The model under review builds one solid part; all positions refer to its coordinate system, in mm. A direction names the side the tool comes from. Give positions to 0.01 mm unless a question says otherwise; leave off trailing zeros. Write each loop counter-clockwise with the first axis right and the second up, starting at its lowest first coordinate (ties: lowest second). Pieces come first, ordered by that corner, then holes. Notation, with made-up numbers: (89.25, 60.25) -> (113.25, 60.25) arc R28 ccw to (113.25, 83.25) -> close; hole circle Ø3 at (74.25, 70.25). An arc over 180 degrees is marked (long way). Use CSV: the item, a comma, the result in double quotes.
```python
from build123d import *

# Parameters (mm, degrees)
SKETCH_1_R          = 30
EXTRUDE_1_DEPTH     = 11
EXTRUDE_2_DEPTH     = 4
CUT_EXTRUDE_1_DEPTH = 1.32
SKETCH_8_R          = 2
CUT_EXTRUDE_2_DEPTH = 50.325449821
CHAMFER_2_SIZE      = 2
EXTRUDE_4_DEPTH     = 4


with BuildPart() as part:
    # 草图1 → 凸台-拉伸1 (new body)
    with BuildSketch(Plane(origin=(0, 0, 0), x_dir=(1, 0, 0), z_dir=(0, 1, 0))):
        with Locations(Location((0, 0, 0), (0, 0, 270))):
            Circle(SKETCH_1_R)
    extrude(amount=EXTRUDE_1_DEPTH)

    # 草图3 → 凸台-拉伸2 (add)
    with BuildSketch(Plane.XZ):
        with BuildLine():
            Line((-34, 0), (-30, 0))
            ThreePointArc((-30, 0), (-21.213203436, -21.213203436), (0, -30))
            Line((0, -30), (0, -34))
            ThreePointArc((0, -34), (-24.04163056, -24.04163056), (-34, 0))
        make_face()
        with BuildLine():
            Line((0, 34), (0, 30))
            ThreePointArc((0, 30), (21.213203436, 21.213203436), (30, 0))
            Line((30, 0), (34, 0))
            ThreePointArc((34, 0), (24.04163056, 24.04163056), (0, 34))
        make_face()
    extrude(amount=-EXTRUDE_2_DEPTH)

    # 草图6 → 切除-旋转8 (revolve, cut)
    with BuildSketch(Plane(origin=(0, 0, 0), x_dir=(-1, 0, 0), z_dir=(0, 0, -1)), mode=Mode.PRIVATE) as cut_revolve_8_sk:
        Polygon((-30, 2.2), (-32, 2.2), (-32, 3.52), (-34, 3.52), (-34, 4), (-30, 4), align=None)
    revolve(cut_revolve_8_sk.sketch.rotate(Axis((0, 0, 0), (0, 1, 0)), 270), axis=Axis((0, 0, 0), (0, 1, 0)), mode=Mode.SUBTRACT)

    # 草图7 → 切除-拉伸1 (cut)
    with BuildSketch(Plane(origin=(0, 3.52, 0), x_dir=(1, 0, 0), z_dir=(0, 1, 0))):
        with BuildLine():
            Line((6.522408084, -31.328233158), (-2.191886095, -31.444458777))
            Line((-2.191886095, -31.444458777), (0, -34))
            ThreePointArc((0, -34), (3.348762467, -32.877867185), (6.522408084, -31.328233158))
        make_face()
        with BuildLine():
            Line((-6.522408084, 31.328233158), (2.581044054, 31.031256101))
            Line((2.581044054, 31.031256101), (0, 34))
            ThreePointArc((0, 34), (-3.348762467, 32.877867185), (-6.522408084, 31.328233158))
        make_face()
    extrude(amount=-CUT_EXTRUDE_1_DEPTH, mode=Mode.SUBTRACT)

    # 草图8 → 切除-拉伸2 (cut, through all)
    with BuildSketch(Plane(origin=(0, 11, 0), x_dir=(1, 0, 0), z_dir=(0, 1, 0))):
        with BuildLine():
            ThreePointArc((14.5, 12.5), (13.914213562, 13.914213562), (12.5, 14.5))
            Line((12.5, 14.5), (12.5, 10.5))
            ThreePointArc((12.5, 10.5), (13.914213562, 11.085786438), (14.5, 12.5))
        make_face()
        with BuildLine():
            Line((12.5, 10.5), (12.5, 14.5))
            ThreePointArc((12.5, 14.5), (10.5, 12.5), (12.5, 10.5))
        make_face()
        with BuildLine():
            ThreePointArc((-12.5, -10.5), (-13.914213562, -11.085786438), (-14.5, -12.5))
            Line((-14.5, -12.5), (-12.5, -12.5))
            Line((-12.5, -12.5), (-12.5, -10.5))
        make_face()
        with BuildLine():
            Line((-12.5, -12.5), (-14.5, -12.5))
            ThreePointArc((-14.5, -12.5), (-13.914213562, -13.914213562), (-12.5, -14.5))
            Line((-12.5, -14.5), (-12.5, -12.5))
        make_face()
        with BuildLine():
            ThreePointArc((-10.5, -12.5), (-11.085786438, -11.085786438), (-12.5, -10.5))
            Line((-12.5, -10.5), (-12.5, -12.5))
            Line((-12.5, -12.5), (-10.5, -12.5))
        make_face()
        with BuildLine():
            Line((-10.5, -12.5), (-12.5, -12.5))
            Line((-12.5, -12.5), (-12.5, -14.5))
            ThreePointArc((-12.5, -14.5), (-11.085786438, -13.914213562), (-10.5, -12.5))
        make_face()
        with Locations(Location((12.5, -12.5, 0), (0, 0, 270))):
            Circle(SKETCH_8_R)
        with Locations(Location((-12.5, 12.5, 0), (0, 0, 270))):
            Circle(SKETCH_8_R)
    extrude(amount=-CUT_EXTRUDE_2_DEPTH, mode=Mode.SUBTRACT)

    # 倒角2
    chamfer_2_edges = [part.edges().sort_by_distance(p)[0] for p in [
        (-12.5, 11, -14.5),
        (12.5, 11, 10.5),
        (-12.5, 11, 10.5),
        (12.5, 11, -14.5),
    ]]
    chamfer(chamfer_2_edges, length=CHAMFER_2_SIZE)

    # 草图13 → 凸台-拉伸4 (add)
    with BuildSketch(Plane(origin=(0, 11, 0), x_dir=(1, 0, 0), z_dir=(0, 1, 0))):
        with BuildLine():
            Line((-3.896027989, 17.813244072), (-9.5, 0))
            Line((-9.5, 0), (-3.797777246, -18.190499049))
            ThreePointArc((-3.797777246, -18.190499049), (0, -20.98), (3.797777246, -18.190499049))
            Line((3.797777246, -18.190499049), (9.5, 0))
            Line((9.5, 0), (3.797777247, 18.190499048))
            ThreePointArc((3.797777247, 18.190499048), (0.198983725, 20.975022701), (-3.659900167, 18.563819291))
            Line((-3.659900167, 18.563819291), (-3.896027989, 17.813244072))
        make_face()
        with BuildLine():
            Line((-1.889470191, -17.591863495), (-7.4, 0))
            Line((-7.4, 0), (-1.889470192, 17.591863494))
            ThreePointArc((-1.889470192, 17.591863494), (0, 18.979999999), (1.889470191, 17.591863494))
            Line((1.889470191, 17.591863494), (7.4, 0))
            Line((7.4, 0), (1.889470191, -17.591863495))
            ThreePointArc((1.889470191, -17.591863495), (0, -18.98), (-1.889470191, -17.591863495))
        make_face(mode=Mode.SUBTRACT)
    extrude(amount=EXTRUDE_4_DEPTH)


solid = part.part
```
Q1. The part is to be moulded in two halves that separate along X. For faces 1 (the cylindrical face through (0.27, 12.97, -20.97)), 2 (the flat face through (0, 1, -32)), 3 (the flat face through (-7, 15, -2)), 4 (the cylindrical face through (14.483, 4.563, 12.24)), say which applies: pulls with the +X half, pulls with the -X half, needs draft (parallel to the pull), parting line crosses it, or undercut.
Derived:
face 1,"parting line crosses it"
face 2,"pulls with the +X half"
face 3,"needs draft"
face 4,"undercut"
Q2. Consider section A-A (y = 7). Write out the cut boundary in (x, z).
Derived:
outline,"circle Ø60 at (0, 0); hole circle Ø4 at (-12.5, -12.5); hole circle Ø4 at (-12.5, 12.5); hole circle Ø4 at (12.5, -12.5); hole circle Ø4 at (12.5, 12.5)"
Q3. Consider section C-C (x = 18.5). Write out the cut boundary in (y, z), then the cut area to 3 significant figures.
Derived:
outline,"(0, -23.62) -> (11, -23.62) -> (11, 23.62) -> (2.2, 23.62) -> (2.2, 26.11) -> (3.52, 26.11) -> (3.52, 28.53) -> (0, 28.53) -> close"
area,"534 mm2"
Q4. Machinability: for faces 5 (the flat face through (-4.606, 12.972, 8.919)), 6 (the flat face through (-6.69, 12.97, 8.97)), 7 (the flat face through (23.4, 3.52, 22.1)), which of the approach directions +Z, -Z, +X, -X, +Y, -Y give a long, thin tool a straight path to every point of the face, cutting with its end or side? Answer none if there is none.
Derived:
face 5,"+Y"
face 6,"+Z, -X, +Y"
face 7,"+Z, +X, +Y"
Q5. To check wall thickness, follow probe 1 along X at (y, z) = (4.75, 12.5); probe 2 along X at (y, z) = (2.75, -12.5); probe 3 along Y at (x, z) = (12.5, -6). State the ranges of each line that lie inside material, in increasing order.
Derived:
probe 1,"x = -27.27 to -14.5, -10.5 to 10.5, 14.5 to 27.27"
probe 2,"x = -31.62 to -29.46, -27.27 to -14.5, -10.5 to 10.5, 14.5 to 27.27"
probe 3,"y = 0 to 11"
Q6. Insertion check: pin 1 (6 mm diameter, centred on y = 11.5, z = -1.5, fed in from +X); pin 2 (2 mm diameter, centred on x = -2.5, y = 12.5, fed in from -Z); pin 3 (1.1 mm diameter, centred on y = 1, z = 32.5, fed in from -X); pin 4 (3 mm diameter, centred on x = 12.5, z = 12.5, fed in from +Y). Each pin has a flat end and moves straight along its axis. Give the tip position at first contact, or say it passes through.
Derived:
pin 1,"stops at x = 30"
pin 2,"stops at z = -20.69"
pin 3,"stops at x = 0"
pin 4,"passes through"
Q7. Consider section B-B (y = 12.5). Write out the cut boundary in (x, z), then the cut area to 3 significant figures.
Derived:
outline,"(-9.5, 0) -> (-3.66, -18.56) arc R3.98 ccw to (3.8, -18.19) -> (9.5, 0) -> (3.8, 18.19) arc R3.98 ccw to (-3.8, 18.19) -> close; hole (-7.4, 0) -> (-1.89, -17.59) arc R1.98 ccw to (1.89, -17.59) -> (7.4, 0) -> (1.89, 17.59) arc R1.98 ccw to (-1.89, 17.59) -> close"
area,"180 mm2"
